```python
from build123d import *

# Parameters (mm, degrees)
SKETCH1_W               = 42
SKETCH1_H               = 40
BOSS_EXTRUDE1_DEPTH     = 25
SKETCH2_R               = 4.45
SKETCH2_W               = 30
SKETCH2_H               = 11.2
CUT_EXTRUDE1_DEPTH      = 25
SKETCH5_W               = 37
SKETCH5_H               = 12.4
CUT_EXTRUDE3_DEPTH      = 23.95
SKETCH7_W               = 5
SKETCH7_H               = 40
BOSS_EXTRUDE2_DEPTH     = 5
SKETCH8_W               = 5
SKETCH8_H               = 40
BOSS_EXTRUDE3_DEPTH     = 5
SKETCH10_W              = 40
SKETCH10_H              = 25
BOSS_EXTRUDE4_DEPTH     = 2.5
CUT_EXTRUDE2_DEPTH      = 66.743841816
CUT_EXTRUDE2_DEPTH_BACK = 66.743841816


with BuildPart() as part:
    # Sketch1 → Boss-Extrude1 (new body)
    with BuildSketch(Plane(origin=(0, 0, 0), x_dir=(-1, 0, 0), z_dir=(0, 1, 0))):
        with Locations((1.474226804, 20.721649485)):
            Rectangle(SKETCH1_W, SKETCH1_H)
    extrude(amount=BOSS_EXTRUDE1_DEPTH)

    # Sketch2 → Cut-Extrude1 (cut)
    with BuildSketch(Plane(origin=(0, 25, 0), x_dir=(-1, 0, 0), z_dir=(0, 1, 0))):
        with Locations(Location((1.474226804, 31.771649485, 0), (0, 0, 90))):
            Circle(SKETCH2_R)
        with Locations((1.474226804, 11.171649485)):
            Rectangle(SKETCH2_W, SKETCH2_H)
    extrude(amount=-CUT_EXTRUDE1_DEPTH, mode=Mode.SUBTRACT)

    # Sketch5 → Cut-Extrude3 (cut)
    with BuildSketch(Plane.XY.offset(40.721649485)):
        with Locations((-1.474226804, 12.5)):
            Rectangle(SKETCH5_W, SKETCH5_H)
    extrude(amount=-CUT_EXTRUDE3_DEPTH, mode=Mode.SUBTRACT)

    # Sketch7 → Boss-Extrude2 (add)
    with BuildSketch(Plane(origin=(0, 25, 0), x_dir=(-1, 0, 0), z_dir=(0, 1, 0))):
        with Locations((19.974226804, 20.721649485)):
            Rectangle(SKETCH7_W, SKETCH7_H)
        with Locations((-17.025773196, 20.721649485)):
            Rectangle(SKETCH7_W, SKETCH7_H)
    extrude(amount=BOSS_EXTRUDE2_DEPTH)

    # Sketch8 → Boss-Extrude3 (add)
    with BuildSketch(Plane.XZ):
        with Locations((-19.974226804, 20.721649485)):
            Rectangle(SKETCH8_W, SKETCH8_H)
        with Locations((17.025773196, 20.721649485)):
            Rectangle(SKETCH8_W, SKETCH8_H)
    extrude(amount=BOSS_EXTRUDE3_DEPTH)

    # Sketch10 → Boss-Extrude4 (add)
    with BuildSketch(Plane(origin=(19.525773196, 0, 0), x_dir=(0, 0, -1), z_dir=(1, 0, 0))):
        with Locations((-20.721649485, 12.5)):
            Rectangle(SKETCH10_W, SKETCH10_H)
    extrude(amount=BOSS_EXTRUDE4_DEPTH)

    # Sketch3 → Cut-Extrude2 (cut, two sides: drawn at the far end of the back side and taken through both)
    with BuildSketch(Plane.YZ.offset(19.525773196).offset(-CUT_EXTRUDE2_DEPTH_BACK)):
        with BuildLine():
            Line((14.423560576, 13.473803847), (12.5, 15.397364423))
            Line((12.5, 15.397364423), (10.576439424, 13.473803847))
            ThreePointArc((10.576439424, 13.473803847), (12.5, 8.171649485), (14.423560576, 13.473803847))
        make_face()
    extrude(amount=CUT_EXTRUDE2_DEPTH + CUT_EXTRUDE2_DEPTH_BACK, mode=Mode.SUBTRACT)


solid = part.part
```
The model under review builds one solid part; all positions refer to its coordinate system, in mm. A direction names the side the tool comes from. Round coordinates to 2 decimals unless told otherwise and drop trailing zeros. Loops run counter-clockwise (first coordinate to the right, second up) from the corner with the lowest first, then second, coordinate; pieces in that order, holes last. Notation, with made-up numbers: (-9.75, 13) - (-2.75, 13) arc R14 ccw to (-2.75, 39) - close; hole circle Ø6 at (66, 78.5). An arc over 180 degrees is marked (long way). Use a Markdown table: item, result. Add a question column.
Q1. Add section B-B (z = 24). State the section outline as (x, y) points, plus the area to 3 significant figures.
Q2. Add section A-A (x = 6.5). State the section outline as (y, z) points.
Q3. Add section D-D (y = -1.5). State the section outline as (x, z) points, plus the area to 3 significant figures.
Q4. Machinability: for faces 1 (the face through (19.526, 27, 20)), 2 (the face through (-17.474, 27, 20)), 3 (the face through (-1, 0, 25)), 4 (the face through (-1, 22, 16.772)), which of the approach directions +Z, -Z, +X, -X, +Y, -Y give a long, thin tool a straight path to every point of the face, cutting with its end or side? Answer none if there is none.
Q5. Add section C-C (z = 16). State the section outline as (x, y) points, plus the area to 4 significant figures.
Q6. Insertion check: pin 1 Ø10 at (x, z) = (-1.47, 31.77) entering from -Y; pin 2 Ø1.5 at (y, z) = (27, 16.5) entering from +X. Each pin has a flat end and moves straight along its axis. Give the tip position at first contact, or say it passes through.
Q7. For probe 1 along X at (y, z) = (28, 24); probe 2 along Z at (x, y) = (-12, 21); probe 3 along Y at (x, z) = (7.5, 17), list the stretches that pass through material, from the lowest coordinate up.
Q8. The part is to be moulded in two halves that separate along Y. For faces 5 (the face through (-2, 18.7, 26)), 6 (the face through (-18, 13, 16.772)), 7 (the face through (-20, -5, 21)), 8 (the face through (14.526, 27, 20)), say which applies: pulls with the +Y half, pulls with the -Y half, needs draft (parallel to the pull), parting line crosses it, or undercut.
Worked answers:
| question | item | result |
|---|---|---|
| 1 | outline | (-22.47, -5) - (-17.47, -5) - (-17.47, 0) - (14.53, 0) - (14.53, -5) - (19.53, -5) - (19.53, 0) - (22.03, 0) - (22.03, 25) - (19.53, 25) - (19.53, 30) - (14.53, 30) - (14.53, 25) - (-17.47, 25) - (-17.47, 30) - (-22.47, 30) - close; hole (-19.97, 6.3) - (17.03, 6.3) - (17.03, 18.7) - (-19.97, 18.7) - close |
| 1 | area | 754 mm² |
| 2 | outline | (0, 0.72) - (25, 0.72) - (25, 5.57) - (0, 5.57) - close; (0, 16.77) - (6.3, 16.77) - (6.3, 40.72) - (0, 40.72) - close; (18.7, 16.77) - (25, 16.77) - (25, 40.72) - (18.7, 40.72) - close |
| 3 | outline | (-22.47, 0.72) - (-17.47, 0.72) - (-17.47, 40.72) - (-22.47, 40.72) - close; (14.53, 0.72) - (19.53, 0.72) - (19.53, 40.72) - (14.53, 40.72) - close |
| 3 | area | 400 mm² |
| 4 | face 1 | +Z, -Z, +X, +Y |
| 4 | face 2 | +Z, -Z, +Y |
| 4 | face 3 | +Z, -Z, -Y |
| 4 | face 4 | +Y, -Y |
| 5 | outline | (-22.47, -5) - (-17.47, -5) - (-17.47, 0) - (-16.47, 0) - (-16.47, 25) - (-17.47, 25) - (-17.47, 30) - (-22.47, 30) - close; (13.53, 0) - (14.53, 0) - (14.53, -5) - (19.53, -5) - (19.53, 0) - (22.03, 0) - (22.03, 25) - (19.53, 25) - (19.53, 30) - (14.53, 30) - (14.53, 25) - (13.53, 25) - close |
| 5 | area | 462.5 mm² |
| 6 | pin 1 | y = 0 |
| 6 | pin 2 | x = 19.53 |
| 7 | probe 1 | -22.47 to -17.47, 14.53 to 19.53 |
| 7 | probe 2 | 0.72 to 5.57, 16.77 to 40.72 |
| 7 | probe 3 | 0 to 6.3, 18.7 to 25 |
| 8 | face 5 | undercut |
| 8 | face 6 | undercut |
| 8 | face 7 | pulls with the -Y half |
| 8 | face 8 | needs draft |
